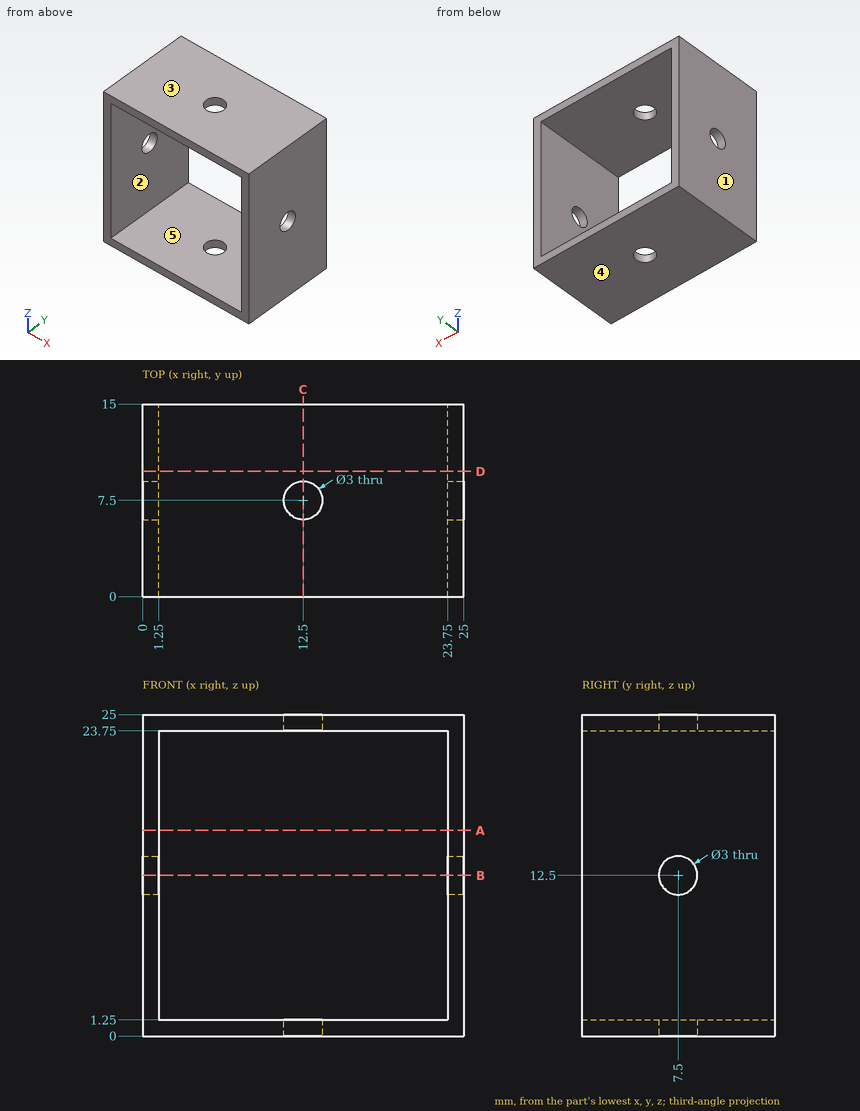
Can you work these out from the drawing? Everything is in mm from the part's minimum corner. A direction names the side the tool comes from. Coordinates: 2 decimals unless noted, no trailing zeros. Loops run counter-clockwise (first coordinate to the right, second up) from the corner with the lowest first, then second, coordinate; pieces in that order, holes last. Notation, with made-up numbers: M -16.75,-21 L 31.25,-21 A16 cw 31.25,4 Z; hole C -3,60 d11. An arc over 180 degrees is marked long. Put each result on its own line as item: value. Start each with the question number.
(1) I need wall thicknesses on line 1 (Z direction, x = 1.5, y = 3); line 2 (Y direction, x = 12.5, z = 24.45). Which ranges of each line are inside material? Lowest first, please. Write a range as from..to.
(2) For the marked faces 1 and 2, which set-ups out of +Z, -Z, +X, -X, +Y, -Y let a thin tool reach every point of the face, with its end or its side?
(3) Thinking about a two-plate mould opening in Z: for the marked faces 3, 4 and 5, which applies, pulls with the +Z half, pulls with the -Z half, needs draft (parallel to the pull), parting line crosses it, or undercut?
(4) Suppose I cut it at B-B on z = 12.5. Please give me the cut outline in (x, y).
(5) Suppose I cut it at C-C on x = 12.5. Please give me the cut outline in (y, z).
(6) Suppose I cut it at D-D on y = 9.75. Please give me the cut outline in (x, z), then the cut area to 3 significant figures.
(7) Suppose I cut it at A-A on z = 16. Please give me the cut outline in (x, y).
Solutions:
1. line 1: z = 0..1.25, 23.75..25
1. line 2: y = 0..6, 9..15
2. face 1: +Z, -Z, -X, +Y, -Y
2. face 2: +Y, -Y
3. face 3: pulls with the +Z half
3. face 4: pulls with the -Z half
3. face 5: undercut
4. outline: M 0,0 L 1.25,0 L 1.25,6 L 0,6 Z; M 0,9 L 1.25,9 L 1.25,15 L 0,15 Z; M 23.75,0 L 25,0 L 25,6 L 23.75,6 Z; M 23.75,9 L 25,9 L 25,15 L 23.75,15 Z
5. outline: M 0,0 L 6,0 L 6,1.25 L 0,1.25 Z; M 0,23.75 L 6,23.75 L 6,25 L 0,25 Z; M 9,0 L 15,0 L 15,1.25 L 9,1.25 Z; M 9,23.75 L 15,23.75 L 15,25 L 9,25 Z
6. outline: M 0,0 L 25,0 L 25,25 L 0,25 Z; hole M 1.25,1.25 L 23.75,1.25 L 23.75,23.75 L 1.25,23.75 Z
6. area: 119 mm2
7. outline: M 0,0 L 1.25,0 L 1.25,15 L 0,15 Z; M 23.75,0 L 25,0 L 25,15 L 23.75,15 Z
